Here's how the part is built. I have some questions about the finished solid (model axes, mm). Round coordinates to 2 decimals unless told otherwise and drop trailing zeros. Write each loop counter-clockwise with the first axis right and the second up, starting at its lowest first coordinate (ties: lowest second). Pieces come first, ordered by that corner, then holes. Notation, with made-up numbers: (40.5, -31.5) -> (75.5, -31.5) arc R29 cw to (75.5, 3.5) -> close; hole circle Ø1 at (-19.75, 75). An arc over 180 degrees is marked (long way). Answer in a Markdown table with one row per item. Add a question column.
from build123d import *

# Parameters (mm, degrees)
SKETCH9_W                              = 19.05
SKETCH9_H                              = 12.7
BOSS_EXTRUDE1_DEPTH                    = 25.4
CUT_EXTRUDE1_DEPTH                     = 27.820764344
SKETCH11_R                             = 4.7625
SKETCH11_R_2                           = 3.175
BOSS_EXTRUDE2_DEPTH                    = 1.5875
F_97_0_0059_DIAMETER_HOLE1_D           = 0.14986
F_97_0_0059_DIAMETER_HOLE1_CSINK_D     = 3.0226
F_97_0_0059_DIAMETER_HOLE1_CSINK_ANGLE = 100


with BuildPart() as part:
    # Sketch9 → Boss-Extrude1 (new body)
    with BuildSketch(Plane(origin=(0, -7.62, 0), x_dir=(1, 0, 0), z_dir=(0, 1, 0))):
        Rectangle(SKETCH9_W, SKETCH9_H)
    extrude(amount=BOSS_EXTRUDE1_DEPTH)

    # Sketch10 → Cut-Extrude1 (cut, through all)
    with BuildSketch(Plane(origin=(9.525, 0, 0), x_dir=(0, 0, -1), z_dir=(1, 0, 0))):
        Polygon((6.35, -7.62), (-6.35, -0.287651581), (-6.35, 22.86), (6.35, 22.86), align=None)
    extrude(amount=-CUT_EXTRUDE1_DEPTH, mode=Mode.SUBTRACT)

    # Sketch11 → Boss-Extrude2 (add)
    with BuildSketch(Plane(origin=(0, -2.965369343, 1.712056788), x_dir=(1, 0, 0), z_dir=(0, 0.8660254037844382, -0.500000000000001))):
        with Locations(Location((0, 0, 0), (0, 0, 270))):
            Circle(SKETCH11_R)
        with Locations(Location((0, 0, 0), (0, 0, 270))):
            Circle(SKETCH11_R_2, mode=Mode.SUBTRACT)
    extrude(amount=BOSS_EXTRUDE2_DEPTH)

    # #97 (0.0059) Diameter Hole1 (through all)
    with Locations(Plane(origin=(0, -7.62, 0), x_dir=(-1, 0, 0), z_dir=(0, -1, 0))):
        with Locations((4.7625, 0), (-4.7625, 0)):
            CounterSinkHole(F_97_0_0059_DIAMETER_HOLE1_D / 2, F_97_0_0059_DIAMETER_HOLE1_CSINK_D / 2, counter_sink_angle=F_97_0_0059_DIAMETER_HOLE1_CSINK_ANGLE)


solid = part.part
Item 1: If we section it at C-C on x = -7.75: Please give me the cut outline in (y, z).
Item 2: If we section it at A-A on x = 1: Please give me the cut outline in (y, z), then the cut area to 3 significant figures.
Item 3: If we mould it in two halves opening along Z, with no side actions, what happens to faces 1 (the flat face through (0.04, -2.99, 1.67)), 2 (the flat face through (0, -4, 6.35)), 3 (the flat face through (-9.525, -5, 2)), 4 (the conical face through (4.52, -6.61, 0.19))? For each: pulls with the +Z half, pulls with the -Z half, needs draft (parallel to the pull), parting line crosses it, or undercut.
Item 4: I need wall thicknesses on line 1 along Z through (x, y) = (5.75, -6.75); line 2 along X through (y, z) = (-2, 2); line 3 along Z through (x, y) = (-3.5, -6.25). Which ranges of each line are inside material? Lowest first, please. Write a range as from..to.
Item 5: For P1, Ø6, axis at x = 0.5, z = 1, coming from the +Y side; P2, Ø1.5, axis at x = 1, y = -4.5, coming from the -Z side, each with a flat end and sliding along its axis, tell me the tip position at first contact or that it passes through.
Item 6: If we section it at B-B on z = -5.5: Please give me the cut outline in (x, y) (3 decimals), then the cut area to 3 significant figures.
Results list:
| question | item | result |
|---|---|---|
| 1 | outline | (-7.62, -6.35) -> (-0.29, 6.35) -> (-7.62, 6.35) -> close |
| 2 | outline | (-7.62, -6.35) -> (-5.29, -2.32) -> (-3.92, -3.11) -> (-3.1, -1.69) -> (-4.47, -0.9) -> (-1.46, 4.32) -> (-0.08, 3.53) -> (0.74, 4.95) -> (-0.64, 5.74) -> (-0.29, 6.35) -> (-7.62, 6.35) -> close |
| 2 | area | 51.8 mm² |
| 3 | face 1 | undercut |
| 3 | face 2 | pulls with the +Z half |
| 3 | face 3 | needs draft |
| 3 | face 4 | undercut |
| 4 | line 1 | -4.84..6.35 |
| 4 | line 2 | -4.71..-3.09, 3.09..4.71 |
| 4 | line 3 | -3.98..6.35 |
| 5 | P1 | y = 0.19 |
| 5 | P2 | z = -3.19 |
| 6 | outline | (-9.525, -7.62) -> (9.525, -7.62) -> (9.525, -7.129) -> (-9.525, -7.129) -> close |
| 6 | area | 9.35 mm² |
